Read the model definition and answer for the solid it produces. Units are mm, in the model's axes. Face numbers are marked on the shaded views. A direction names the side the tool comes from. Coordinates: 2 decimals unless noted, no trailing zeros. Loops run counter-clockwise (first coordinate to the right, second up) from the corner with the lowest first, then second, coordinate; pieces in that order, holes last. Notation, with made-up numbers: (-24.5, 11.25) - (23.5, 11.25) arc R8 ccw to (23.5, 21.25) - close; hole circle Ø1 at (30, -3.5). An arc over 180 degrees is marked (long way). Use one line per item in the form item = value.
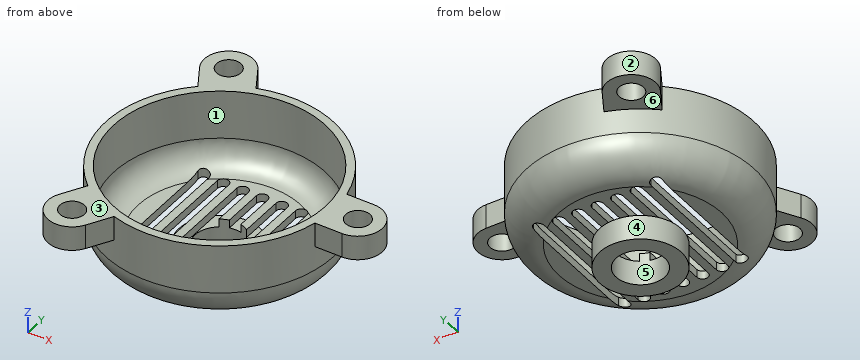
from build123d import *

# Parameters (mm, degrees)
SKETCH1_R               = 3.5
BOSS_EXTRUDE1_DEPTH     = 1.25
FILLET1_R               = 1
SHELL1_T                = -0.25
CUT_EXTRUDE1_DEPTH      = 6.545268253
LPATTERN1_COUNT         = 4
LPATTERN1_PITCH         = 0.6
LPATTERN2_COUNT         = 4
LPATTERN2_PITCH         = 0.6
SKETCH3_R               = 1.25
BOSS_EXTRUDE2_DEPTH     = 0.75
CUT_EXTRUDE2_DEPTH      = 6.545268379
CUT_EXTRUDE2_DEPTH_BACK = 6.545268379
SKETCH3_3_R             = 0.75
SKETCH4_R               = 0.375
BOSS_EXTRUDE3_DEPTH     = 0.75
CIRPATTERN1_COUNT       = 3


with BuildPart() as part:
    # Sketch1 → Boss-Extrude1 (new, symmetric)
    with BuildSketch(Plane.XY):
        Circle(SKETCH1_R)
    extrude(amount=BOSS_EXTRUDE1_DEPTH, both=True)

    # Fillet1
    fillet1_edges = [part.edges().sort_by_distance(p)[0] for p in [
        (-3.5, 0, -1.25),
    ]]
    fillet(fillet1_edges, radius=FILLET1_R)

    # Shell1
    shell1_openings = [part.faces().sort_by_distance(p)[0] for p in [
        (0, 0, 1.25),
    ]]
    offset(amount=SHELL1_T, openings=shell1_openings, kind=Kind.INTERSECTION)

    # Sketch2 → Cut-Extrude1 (cut, through all)
    with BuildSketch(Plane(origin=(0, 0, -1.25), x_dir=(-1, 0, 0), z_dir=(0, 0, -1))):
        with BuildLine():
            Line((0.175, 2), (0.175, -2))
            ThreePointArc((0.175, -2), (0, -2.175), (-0.175, -2))
            Line((-0.175, -2), (-0.175, 2))
            ThreePointArc((-0.175, 2), (0, 2.175), (0.175, 2))
        make_face()
    cut_extrude1 = extrude(amount=-CUT_EXTRUDE1_DEPTH, mode=Mode.SUBTRACT)

    # LPattern1: Cut-Extrude1 ×4
    with Locations(*[(i * LPATTERN1_PITCH, 0, 0) for i in range(1, LPATTERN1_COUNT)]):
        add(cut_extrude1, mode=Mode.SUBTRACT)

    # LPattern2: Cut-Extrude1 ×4
    with Locations(*[(-i * LPATTERN2_PITCH, 0, 0) for i in range(1, LPATTERN2_COUNT)]):
        add(cut_extrude1, mode=Mode.SUBTRACT)

    # Sketch3 → Boss-Extrude2 (add)
    with BuildSketch(Plane(origin=(0, 0, -1.25), x_dir=(-1, 0, 0), z_dir=(0, 0, -1))):
        with Locations(Location((0, 0, 0), (0, 0, 145.084793753))):
            Circle(SKETCH3_R)
    extrude(amount=BOSS_EXTRUDE2_DEPTH)

    # Sketch3_3 → Cut-Extrude2 (cut, two sides: drawn at the far end of the back side and taken through both)
    with BuildSketch(Plane(origin=(0, 0, -1.25), x_dir=(-1, 0, 0), z_dir=(0, 0, -1)).offset(-CUT_EXTRUDE2_DEPTH_BACK)):
        Circle(SKETCH3_3_R)
    extrude(amount=CUT_EXTRUDE2_DEPTH + CUT_EXTRUDE2_DEPTH_BACK, mode=Mode.SUBTRACT)

    # Sketch4 → Boss-Extrude3 (add)
    with BuildSketch(Plane.XY.offset(1.25)):
        with BuildLine():
            Line((4.25, 0.75), (3.418698583, 0.75))
            ThreePointArc((3.418698583, 0.75), (3.5, 0), (3.418698583, -0.75))
            Line((3.418698583, -0.75), (4.25, -0.75))
            ThreePointArc((4.25, -0.75), (5, 0), (4.25, 0.75))
        make_face()
        with Locations((4.25, 0)):
            Circle(SKETCH4_R, mode=Mode.SUBTRACT)
    boss_extrude3 = extrude(amount=-BOSS_EXTRUDE3_DEPTH)

    # CirPattern1: Boss-Extrude3 ×3 about axis
    cirpattern1_axis = Axis((0, 0, 0), (0, 0, 1))
    for i in range(1, CIRPATTERN1_COUNT):
        add(boss_extrude3.rotate(cirpattern1_axis, i * 360 / CIRPATTERN1_COUNT))


solid = part.part
Item 1: Find the intervals of material crossed by L1, parallel to X at y = 0, z = -1.5; L2, parallel to Y at x = -2.25, z = 0.85; L3, parallel to Y at x = -2.75, z = 0.9, in increasing order.
Results below:
L1 = -1.25 to -0.75, 0.75 to 1.25
L2 = -4.42 to -4.03, -3.33 to -2.35, 2.35 to 3.33, 4.03 to 4.42
L3 = -4.1 to -3.26, -2.17 to -1.73, 1.73 to 2.17, 3.26 to 4.1
Item 2: The part is cut by section B-B on z = -1.7. Give the vertices of the cut face in (x, y) (3 decimals), plus the area to 3 significant figures.
Results below:
outline = circle Ø2.5 at (0, 0); hole circle Ø1.5 at (0, 0)
area = 3.14 mm²
Item 3: The part is cut by section A-A on y = 0. Count the separate pieces of the cut face and the enclosed holes in it, plus the area to 3 significant figures.
Results below:
separate_pieces = 7
enclosed_holes = 0
area = 3.26 mm²
Item 4: Each of these flat-tipped pins is pushed along its axis until it touches: P1, Ø2, axis at x = -2, y = -3.5, coming from the -Z side; P2, Ø1, axis at x = 1, z = -0.5, coming from the +Y side; P3, Ø1.4, axis at x = 0, y = -2, coming from the -Z side. Where does it stop, or does it pass through?
Results below:
P1 = -1.1
P2 = 3.46
P3 = -1.25
Item 5: Which of the six approach directions +Z, -Z, +X, -X, +Y, -Y give full straight-line access (tool end or side, diameter ignored) to the marked faces 4, 5 and 6?
Results below:
face_4 = -Z
face_5 = +Z, -Z
face_6 = -Z, -X, +Y
Item 6: For a pull along X with two mould halves and no side action, classify the marked faces 1, 2 and 3 as +X half, -X half, draft (parallel to the pull), parting line (faces both ways), or undercut.
Results below:
face_1 = undercut
face_2 = parting line
face_3 = draft
